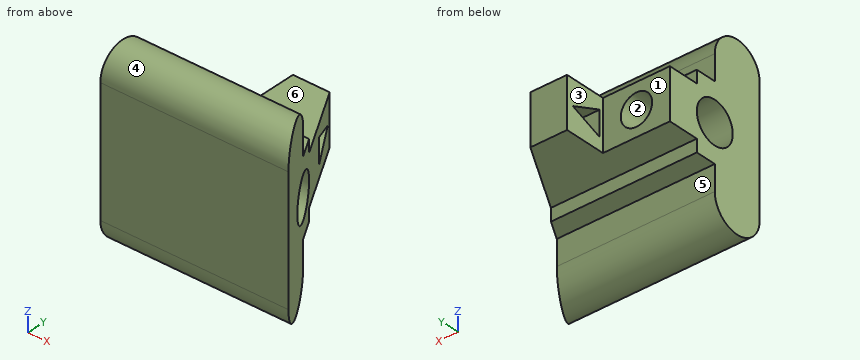
from build123d import *

# Parameters (mm, degrees)
SKETCH3_W               = 24
SKETCH3_H               = 35
BOSS_EXTRUDE1_DEPTH     = 90
SKETCH4_R               = 10
CUT_EXTRUDE1_DEPTH      = 91
SKETCH6_W               = 32
SKETCH6_H               = 24
CUT_EXTRUDE2_DEPTH      = 20
CUT_EXTRUDE4_REACH      = 52
SKETCH7_R               = 7.5
CUT_EXTRUDE5_DEPTH      = 31.5
CUT_EXTRUDE5_DEPTH_BACK = 55.5
CUT_EXTRUDE6_REACH      = 92


with BuildPart() as part:
    # Sketch3 → Boss-Extrude1 (new body)
    with BuildSketch(Plane(origin=(0, 0, 0), x_dir=(0, 0, -1), z_dir=(1, 0, 0))):
        with BuildLine():
            Line((-30, -12.5), (30, -12.5))
            ThreePointArc((30, -12.5), (42.5, 0), (30, 12.5))
            Line((30, 12.5), (-30, 12.5))
            ThreePointArc((-30, 12.5), (-42.5, 0), (-30, -12.5))
        make_face()
        Polygon((-18, 22.5), (-18, 12.5), (18, 12.5), (18, 22.5), (12, 22.5), (-12, 22.5), align=None)
        with Locations((0, 40)):
            Rectangle(SKETCH3_W, SKETCH3_H)
    extrude(amount=BOSS_EXTRUDE1_DEPTH)

    # Sketch4 → Cut-Extrude1 (cut, through all)
    with BuildSketch(Plane(origin=(90, 0, 0), x_dir=(0, 0, -1), z_dir=(1, 0, 0))):
        with Locations((0, 12.5)):
            Circle(SKETCH4_R)
    extrude(amount=-CUT_EXTRUDE1_DEPTH, mode=Mode.SUBTRACT)

    # Sketch6 → Cut-Extrude2 (cut)
    with BuildSketch(Plane(origin=(0, 57.5, 0), x_dir=(1, 0, 0), z_dir=(0, 1, 0))):
        with Locations((16, 0)):
            Rectangle(SKETCH6_W, SKETCH6_H)
    extrude(amount=-CUT_EXTRUDE2_DEPTH, mode=Mode.SUBTRACT)

    # Sketch7 → Cut-Extrude4 (cut, up to next)
    with BuildSketch(Plane(origin=(0, 37.5, 0), x_dir=(1, 0, 0), z_dir=(0, 1, 0)), mode=Mode.PRIVATE) as cut_extrude4_sk1:
        with Locations((16, 0)):
            Circle(SKETCH7_R)
    cut_extrude4_tool1 = extrude(cut_extrude4_sk1.sketch, amount=-CUT_EXTRUDE4_REACH, mode=Mode.PRIVATE) & part.part
    add(cut_extrude4_tool1.solids().sort_by_distance((16, 37.5, 0))[0], mode=Mode.SUBTRACT)

    # Sketch9 → Cut-Extrude5 (cut, two sides)
    with BuildSketch(Plane.XY.offset(12)) as cut_extrude5_sk:
        Polygon((90, 22.5), (90, 57.5), (49.585481157, 57.5), (90, -12.5), (90, 12.5), align=None)
    extrude(amount=CUT_EXTRUDE5_DEPTH, mode=Mode.SUBTRACT)
    extrude(cut_extrude5_sk.sketch, amount=-CUT_EXTRUDE5_DEPTH_BACK, mode=Mode.SUBTRACT)

    # Sketch15 → Cut-Extrude6 (cut, up to next)
    with BuildSketch(Plane(origin=(90, 0, 0), x_dir=(0, 0, -1), z_dir=(1, 0, 0)), mode=Mode.PRIVATE) as cut_extrude6_sk1:
        Polygon((0, 54.316366077), (-6, 39.316366077), (6, 39.316366077), align=None)
    cut_extrude6_tool1 = extrude(cut_extrude6_sk1.sketch, amount=-CUT_EXTRUDE6_REACH, mode=Mode.PRIVATE) & part.part
    add(cut_extrude6_tool1.solids().sort_by_distance((90, 44.316366, 0))[0], mode=Mode.SUBTRACT)


solid = part.part
CAD build for the part. Positions are in the model's coordinates, mm. Face numbers are marked on the shaded views. A direction names the side the tool comes from. Give positions to 0.01 mm unless a question says otherwise; leave off trailing zeros. Loops run counter-clockwise (first coordinate to the right, second up) from the corner with the lowest first, then second, coordinate; pieces in that order, holes last. Notation, with made-up numbers: M 58,66 L 63,66 A12 cw 63,80 Z; hole C -29.75,11 d9. An arc over 180 degrees is marked long. Answer in a Markdown table with one row per item. Add a question column.
Item 1: Mould opens along X. For the marked faces 1, 2 and 3 say: +X half, -X half, draft (parallel to the pull), parting line (faces both ways), or undercut.
Item 2: Tool access for the marked faces 4, 5 and 6: list every direction of +Z, -Z, +X, -X, +Y, -Y with a clear straight run to the whole face (end or side of a thin tool).
Item 3: Band-saw the part on C-C on x = 46.5. Give the cut face in (y, z), then the cut area to 3 significant figures.
Item 4: Band-saw the part on A-A on y = 48.5. Give the cut face in (x, z).
Item 5: Drop flat-ended pins along their axis: P1, Ø12, axis at y = 49.5, z = -11.5, coming from the +X side; P2, Ø3, axis at x = 33.5, y = 19.5, coming from the -Z side; P3, Ø11, axis at x = 23, y = 15.5, coming from the +Z side. Give the stop position or say it passes through.
Item 6: Probe probe 1 along Z at (x, y) = (16, 29); probe 2 along Z at (x, y) = (50, 13); probe 3 along Z at (x, y) = (33.5, 34). List the from-to ranges inside material, lowest first.
Item 7: Band-saw the part on B-B on x = 16. Give the cut face in (y, z).
Item 8: Band-saw the part on D-D on z = -4.5. Give the cut face in (x, y), then the cut area to 3 significant figures.
Reply:
| question | item | result |
|---|---|---|
| 1 | face 1 | draft |
| 1 | face 2 | undercut |
| 1 | face 3 | -X half |
| 2 | face 4 | +Z, +X, -X |
| 2 | face 5 | -Z, +X, -X, +Y |
| 2 | face 6 | +Z, +X, -X, +Y |
| 3 | outline | M -12.5,-30 A12.5 ccw 12.5,-30 L 12.5,-18 L 22.5,-18 L 22.5,-12 L 57.5,-12 L 57.5,12 L 22.5,12 L 22.5,18 L 12.5,18 L 12.5,30 A12.5 ccw -12.5,30 Z; hole C 12.5,0 d20; hole M 39.32,-6 L 54.32,0 L 39.32,6 Z |
| 3 | area | 2,790 mm^2 |
| 4 | outline | M 32,-12 L 54.78,-12 L 54.78,-2.33 L 32,-2.33 Z; M 32,2.33 L 54.78,2.33 L 54.78,12 L 32,12 Z |
| 5 | P1 | stops at x = 57.67 |
| 5 | P2 | stops at z = -18 |
| 5 | P3 | stops at z = 37.5 |
| 6 | probe 1 | z = -12 to -7.5, 7.5 to 12 |
| 6 | probe 2 | z = -18 to -9.99, 9.99 to 18 |
| 6 | probe 3 | z = -12 to 12 |
| 7 | outline | M -12.5,-30 A12.5 ccw 12.5,-30 L 12.5,-18 L 22.5,-18 L 22.5,-12 L 37.5,-12 L 37.5,-7.5 L 19.11,-7.5 A10 cw long 19.11,7.5 L 37.5,7.5 L 37.5,12 L 22.5,12 L 22.5,18 L 12.5,18 L 12.5,30 A12.5 ccw -12.5,30 Z |
| 8 | outline | M 0,-12.5 L 90,-12.5 L 80.72,3.57 L 0,3.57 Z; M 0,21.43 L 10,21.43 L 10,37.5 L 0,37.5 Z; M 22,21.43 L 70.41,21.43 L 60.08,39.32 L 32,39.32 L 32,37.5 L 22,37.5 Z; M 32,43.07 L 57.92,43.07 L 49.59,57.5 L 32,57.5 Z |
| 8 | area | 2,600 mm^2 |
